```python
from build123d import *

# Parameters (mm, degrees)
SKETCH_1_W      = 450
SKETCH_1_H      = 40
SKETCH_1_R      = 1.5
SKETCH_1_R_2    = 2
EXTRUDE_1_DEPTH = 5
CHAMFER_1_SIZE  = 2


with BuildPart() as part:
    # 草图1 → 凸台-拉伸1 (new body)
    with BuildSketch(Plane(origin=(0, 0, 0), x_dir=(1, 0, 0), z_dir=(0, 1, 0))):
        Rectangle(SKETCH_1_W, SKETCH_1_H)
        with Locations(Location((215, 12.5, 0), (0, 0, 270))):
            Circle(SKETCH_1_R, mode=Mode.SUBTRACT)
        with Locations(Location((195, 12.5, 0), (0, 0, 270))):
            Circle(SKETCH_1_R, mode=Mode.SUBTRACT)
        with Locations(Location((195, -12.5, 0), (0, 0, 90))):
            Circle(SKETCH_1_R, mode=Mode.SUBTRACT)
        with Locations(Location((215, -12.5, 0), (0, 0, 90))):
            Circle(SKETCH_1_R, mode=Mode.SUBTRACT)
        with Locations(Location((65, -12.5, 0), (0, 0, 90))):
            Circle(SKETCH_1_R, mode=Mode.SUBTRACT)
        with Locations(Location((45, 12.5, 0), (0, 0, 270))):
            Circle(SKETCH_1_R, mode=Mode.SUBTRACT)
        with Locations(Location((65, 12.5, 0), (0, 0, 270))):
            Circle(SKETCH_1_R, mode=Mode.SUBTRACT)
        with Locations(Location((45, -12.5, 0), (0, 0, 90))):
            Circle(SKETCH_1_R, mode=Mode.SUBTRACT)
        with Locations(Location((-210, 10, 0), (0, 0, 270))):
            Circle(SKETCH_1_R_2, mode=Mode.SUBTRACT)
        with Locations(Location((-210, -10, 0), (0, 0, 270))):
            Circle(SKETCH_1_R_2, mode=Mode.SUBTRACT)
    extrude(amount=EXTRUDE_1_DEPTH)

    # 倒角1
    chamfer_1_edges = [part.edges().sort_by_distance(p)[0] for p in [
        (215, 0, -14),
        (195, 0, -14),
        (195, 0, 14),
        (215, 0, 14),
        (65, 0, -14),
        (45, 0, -14),
        (45, 0, 14),
        (65, 0, 14),
    ]]
    chamfer(chamfer_1_edges, length=CHAMFER_1_SIZE)


solid = part.part
```
Geometry: final body of the model. Coordinates: model frame, mm. Coordinates: 2 decimals unless noted, no trailing zeros. Write each question's results on one line, items separated by ' | '. Start each with the question number.
1) Mould query, pull axis X, two halves, no side actions, for faces 1 (the flat face through (-3, 5, 0)), 2 (the conical face through (216.59, 1.87, 12.85)). Classes: released by +X, released by -X, zero draft, split by the parting line, or undercut.
2) Material intervals for line 1 along Z through (x, y) = (195, 3); line 2 along X through (y, z) = (4.1, 12.5); line 3 along X through (y, z) = (4.75, -13), sorted ascending.
3) First-contact query: pin 1 (1.8 mm diameter, centred on x = 215, z = -12.5, fed in from -Y). Flat tip, straight axial feed; report the tip coordinate or a pass-through.
Checks:
1) face 1: zero draft | face 2: undercut
2) line 1: -20 to -14, -11 to 11, 14 to 20 | line 2: -225 to 43.5, 46.5 to 63.5, 66.5 to 193.5, 196.5 to 213.5, 216.5 to 225 | line 3: -225 to 43.59, 46.41 to 63.59, 66.41 to 193.59, 196.41 to 213.59, 216.41 to 225
3) pin 1: through
